from build123d import *

# Parameters (mm, degrees)
SKETCH1_W             = 76.2
SKETCH1_H             = 88.9
BOSS_EXTRUDE1_DEPTH   = 3.175
SKETCH4_W             = 9.144
SKETCH4_H             = 88.9
BOSS_EXTRUDE2_DEPTH   = 6.096
F_6_CLEARANCE_HOLE1_D = 3.7973
SKETCH5_R             = 5.08
BOSS_EXTRUDE3_DEPTH   = 6.096
F_6_CLEARANCE_HOLE2_D = 3.7973


with BuildPart() as part:
    # Sketch1 → Boss-Extrude1 (new body)
    with BuildSketch(Plane(origin=(0, 0, 0), x_dir=(1, 0, 0), z_dir=(0, 1, 0))):
        Rectangle(SKETCH1_W, SKETCH1_H)
    extrude(amount=BOSS_EXTRUDE1_DEPTH)

    # Sketch4 → Boss-Extrude2 (add)
    with BuildSketch(Plane.XZ):
        with Locations((-10.16, 0)):
            Rectangle(SKETCH4_W, SKETCH4_H)
    extrude(amount=BOSS_EXTRUDE2_DEPTH)

    # #6 Clearance Hole1 (through all)
    with Locations(Plane(origin=(-10.16, 3.175, -38.1), x_dir=(0, 0, 1), z_dir=(0, 1, 0))):
        with Locations((0, 0), (76.2, 0)):
            Hole(F_6_CLEARANCE_HOLE1_D / 2)

    # Sketch5 → Boss-Extrude3 (add)
    with BuildSketch(Plane.XZ.offset(6.096)):
        with Locations((-13.01496, 0)):
            Circle(SKETCH5_R)
        with Locations((-13.01496, 21.59)):
            Circle(SKETCH5_R)
        with Locations((-13.01496, -21.59)):
            Circle(SKETCH5_R)
    extrude(amount=-BOSS_EXTRUDE3_DEPTH)

    # #6 Clearance Hole2 (through all)
    with Locations(Plane(origin=(-13.01496, 3.175, 0), x_dir=(0, 0, 1), z_dir=(0, 1, 0))):
        with Locations((0, 0), (-21.59, 0), (21.59, 0)):
            Hole(F_6_CLEARANCE_HOLE2_D / 2)


solid = part.part
Source: CAD feature listing. Evaluate the final solid. Frame: model axes, mm. A direction names the side the tool comes from. Give positions to 0.01 mm unless a question says otherwise; leave off trailing zeros. Order: outer loops, then holes, each group sorted by start corner. A loop starts at its lowest first (then second) coordinate and runs counter-clockwise, first axis right, second up. Notation, with made-up numbers: (79.5, -23.75) -> (138.5, -23.75) arc R15 cw to (138.5, -7.75) -> close; hole circle Ø4 at (73.25, 54). An arc over 180 degrees is marked (long way). Use a Markdown table: item, result.
1) Section query C-C, the plane z = -21.59. Return the cut outline in (x, y) (3 decimals), then the cut area to 3 significant figures.
Answer list:
| item | result |
|---|---|
| outline | (-38.1, 0) -> (-18.095, 0) -> (-18.095, -6.096) -> (-14.914, -6.096) -> (-14.914, 3.175) -> (-38.1, 3.175) -> close; (-11.116, -6.096) -> (-5.588, -6.096) -> (-5.588, 0) -> (38.1, 0) -> (38.1, 3.175) -> (-11.116, 3.175) -> close |
| area | 283 mm² |
2) Ray query, line 1 along X through (y, z) = (-3.5, 0); line 2 along X through (y, z) = (-3, -38.1); line 3 along Z through (x, y) = (-8.5, 0.25). Return the intervals inside material, ascending. Write a range as [from, to].
Answer list:
| item | result |
|---|---|
| line 1 | [-18.09, -14.91], [-11.12, -5.59] |
| line 2 | [-14.73, -12.06], [-8.26, -5.59] |
| line 3 | [-44.45, -39.02], [-37.18, 37.18], [39.02, 44.45] |
3) Mould query, pull axis Z, two halves, no side actions, for faces 4 (the flat face through (16, 0, -1)), 5 (the cylindrical face through (-13.742, -1.525, 19.836)), 6 (the flat face through (-1, 1, 44.45)). Classes: +Z half, -Z half, draft (parallel to the pull), parting line (faces both ways), or undercut.
Answer list:
| item | result |
|---|---|
| face 4 | draft |
| face 5 | undercut |
| face 6 | +Z half |
4) Section query A-A, the plane z = -38.1. Return the cut outline in (x, y) (3 decimals).
Answer list:
| item | result |
|---|---|
| outline | (-38.1, 0) -> (-14.732, 0) -> (-14.732, -6.096) -> (-12.059, -6.096) -> (-12.059, 3.175) -> (-38.1, 3.175) -> close; (-8.261, -6.096) -> (-5.588, -6.096) -> (-5.588, 0) -> (38.1, 0) -> (38.1, 3.175) -> (-8.261, 3.175) -> close |
5) Reachability of faces 1 (the flat face through (-14.732, -3, 35)), 2 (the flat face through (-14.732, -3, -11)), 3 (the flat face through (-14.732, -3, -36)) from +Z, -Z, +X, -X, +Y, -Y: full face, straight path, thin tool, end or side. Return the list, or none.
Answer list:
| item | result |
|---|---|
| face 1 | +Z, -X, -Y |
| face 2 | -X, -Y |
| face 3 | -Z, -X, -Y |
6) Section query B-B, the plane x = -10.16. Return the cut outline in (y, z) (3 decimals).
Answer list:
| item | result |
|---|---|
| outline | (-6.096, -44.45) -> (3.175, -44.45) -> (3.175, -39.999) -> (-6.096, -39.999) -> close; (-6.096, -36.201) -> (3.175, -36.201) -> (3.175, 36.201) -> (-6.096, 36.201) -> close; (-6.096, 39.999) -> (3.175, 39.999) -> (3.175, 44.45) -> (-6.096, 44.45) -> close |
7) Contact query for flat-ended pins moving along their axis: P1, Ø6, axis at x = 25, z = -8, coming from the -Y side; P2, Ø3, axis at y = -2.5, z = -40, coming from the -X side; P3, Ø1.8, axis at y = -3, z = 12, coming from the +X side. Output: stop coordinate, or through.
Answer list:
| item | result |
|---|---|
| P1 | y = 0 |
| P2 | x = -14.73 |
| P3 | x = -5.59 |
8) Section query D-D, the plane y = -1.25. Return the cut outline in (x, z), then the cut area to 3 significant figures.
Answer list:
| item | result |
|---|---|
| outline | (-14.73, -44.45) -> (-5.59, -44.45) -> (-5.59, 44.45) -> (-14.73, 44.45) -> (-14.73, 26.37) arc R5.08 ccw to (-14.73, 16.81) -> (-14.73, 4.78) arc R5.08 ccw to (-14.73, -4.78) -> (-14.73, -16.81) arc R5.08 ccw to (-14.73, -26.37) -> close; hole circle Ø3.8 at (-13.01, -21.59); hole circle Ø3.8 at (-13.01, 0); hole circle Ø3.8 at (-13.01, 21.59); hole circle Ø3.8 at (-10.16, -38.1); hole circle Ø3.8 at (-10.16, 38.1) |
| area | 827 mm² |
